from build123d import *

# Parameters (mm, degrees)
SKETCH1_W           = 101.6
SKETCH1_H           = 38.1
BOSS_EXTRUDE1_DEPTH = 38.1
BOSS_EXTRUDE2_DEPTH = 25.4
BOSS_EXTRUDE3_DEPTH = 381
SCALE1_SCALE        = 1.5


with BuildPart() as part:
    # Sketch1 → Boss-Extrude1 (new body)
    with BuildSketch(Plane(origin=(0, 0, 0), x_dir=(1, 0, 0), z_dir=(0, 1, 0))):
        with Locations((50.8, 19.05)):
            Rectangle(SKETCH1_W, SKETCH1_H)
    extrude(amount=BOSS_EXTRUDE1_DEPTH)

    # Sketch2 → Boss-Extrude2 (add)
    with BuildSketch(Plane(origin=(101.6, 0, 0), x_dir=(0, 0, -1), z_dir=(1, 0, 0))):
        with BuildLine():
            ThreePointArc((28.108587284, 28.108587284), (19.05, 31.860776993), (9.991412716, 28.108587284))
            Line((9.991412716, 28.108587284), (19.05, 19.05))
            Line((19.05, 19.05), (28.108587284, 28.108587284))
        make_face()
        with BuildLine():
            Line((19.05, 19.05), (9.991412716, 28.108587284))
            ThreePointArc((9.991412716, 28.108587284), (6.239223007, 19.05), (9.991412716, 9.991412716))
            Line((9.991412716, 9.991412716), (19.05, 19.05))
        make_face()
        with BuildLine():
            Line((28.108587284, 28.108587284), (19.05, 19.05))
            Line((19.05, 19.05), (28.108587284, 9.991412716))
            ThreePointArc((28.108587284, 9.991412716), (30.885614659, 14.147527889), (31.860776993, 19.05))
            ThreePointArc((31.860776993, 19.05), (30.885614659, 23.952472111), (28.108587284, 28.108587284))
        make_face()
        with BuildLine():
            Line((28.108587284, 9.991412716), (19.05, 19.05))
            Line((19.05, 19.05), (9.991412716, 9.991412716))
            ThreePointArc((9.991412716, 9.991412716), (19.05, 6.239223007), (28.108587284, 9.991412716))
        make_face()
    extrude(amount=BOSS_EXTRUDE2_DEPTH)

    # Sketch3 → Boss-Extrude3 (add)
    with BuildSketch(Plane(origin=(0, 38.1, 0), x_dir=(1, 0, 0), z_dir=(0, 1, 0))):
        with BuildLine():
            Line((33.415123016, 4.684876984), (19.05, 19.05))
            Line((19.05, 19.05), (4.684876984, 4.684876984))
            ThreePointArc((4.684876984, 4.684876984), (8.08545393, 1.947595257), (11.992307848, 0))
            Line((11.992307848, 0), (26.107692152, 0))
            ThreePointArc((26.107692152, 0), (30.01454607, 1.947595257), (33.415123016, 4.684876984))
        make_face()
        with BuildLine():
            Line((33.415123016, 33.415123016), (19.05, 19.05))
            Line((19.05, 19.05), (33.415123016, 4.684876984))
            ThreePointArc((33.415123016, 4.684876984), (37.818937718, 11.275651446), (39.365351794, 19.05))
            ThreePointArc((39.365351794, 19.05), (37.818937718, 26.824348554), (33.415123016, 33.415123016))
        make_face()
        with BuildLine():
            ThreePointArc((11.992307848, 38.1), (8.08545393, 36.152404743), (4.684876984, 33.415123016))
            Line((4.684876984, 33.415123016), (19.05, 19.05))
            Line((19.05, 19.05), (33.415123016, 33.415123016))
            ThreePointArc((33.415123016, 33.415123016), (30.01454607, 36.152404743), (26.107692152, 38.1))
            Line((26.107692152, 38.1), (11.992307848, 38.1))
        make_face()
        with BuildLine():
            Line((19.05, 19.05), (4.684876984, 33.415123016))
            ThreePointArc((4.684876984, 33.415123016), (1.947595257, 30.01454607), (0, 26.107692152))
            Line((0, 26.107692152), (0, 11.992307848))
            ThreePointArc((0, 11.992307848), (1.947595257, 8.08545393), (4.684876984, 4.684876984))
            Line((4.684876984, 4.684876984), (19.05, 19.05))
        make_face()
        with BuildLine():
            ThreePointArc((35.21117424, 35.21117424), (33.516839784, 36.74400046), (31.677929586, 38.1))
            Line((31.677929586, 38.1), (26.107692152, 38.1))
            ThreePointArc((26.107692152, 38.1), (30.01454607, 36.152404743), (33.415123016, 33.415123016))
            Line((33.415123016, 33.415123016), (35.21117424, 35.21117424))
        make_face()
        with BuildLine():
            ThreePointArc((41.905351794, 19.05), (40.165591731, 27.796364472), (35.21117424, 35.21117424))
            Line((35.21117424, 35.21117424), (33.415123016, 33.415123016))
            ThreePointArc((33.415123016, 33.415123016), (37.818937718, 26.824348554), (39.365351794, 19.05))
            ThreePointArc((39.365351794, 19.05), (37.818937718, 11.275651446), (33.415123016, 4.684876984))
            Line((33.415123016, 4.684876984), (35.21117424, 2.88882576))
            ThreePointArc((35.21117424, 2.88882576), (40.165591731, 10.303635528), (41.905351794, 19.05))
        make_face()
        with BuildLine():
            Line((35.21117424, 2.88882576), (33.415123016, 4.684876984))
            ThreePointArc((33.415123016, 4.684876984), (30.01454607, 1.947595257), (26.107692152, 0))
            Line((26.107692152, 0), (31.677929586, 0))
            ThreePointArc((31.677929586, 0), (33.516839784, 1.35599954), (35.21117424, 2.88882576))
        make_face()
        with BuildLine():
            Line((4.684876984, 4.684876984), (2.88882576, 2.88882576))
            ThreePointArc((2.88882576, 2.88882576), (4.583160216, 1.35599954), (6.422070414, 0))
            Line((6.422070414, 0), (11.992307848, 0))
            ThreePointArc((11.992307848, 0), (8.08545393, 1.947595257), (4.684876984, 4.684876984))
        make_face()
        with BuildLine():
            Line((0, 11.992307848), (0, 6.422070414))
            ThreePointArc((0, 6.422070414), (1.35599954, 4.583160216), (2.88882576, 2.88882576))
            Line((2.88882576, 2.88882576), (4.684876984, 4.684876984))
            ThreePointArc((4.684876984, 4.684876984), (1.947595257, 8.08545393), (0, 11.992307848))
        make_face()
        with BuildLine():
            ThreePointArc((6.422070414, 38.1), (4.583160216, 36.74400046), (2.88882576, 35.21117424))
            Line((2.88882576, 35.21117424), (4.684876984, 33.415123016))
            ThreePointArc((4.684876984, 33.415123016), (8.08545393, 36.152404743), (11.992307848, 38.1))
            Line((11.992307848, 38.1), (6.422070414, 38.1))
        make_face()
        with BuildLine():
            Line((4.684876984, 33.415123016), (2.88882576, 35.21117424))
            ThreePointArc((2.88882576, 35.21117424), (1.35599954, 33.516839784), (0, 31.677929586))
            Line((0, 31.677929586), (0, 26.107692152))
            ThreePointArc((0, 26.107692152), (1.947595257, 30.01454607), (4.684876984, 33.415123016))
        make_face()
    extrude(amount=BOSS_EXTRUDE3_DEPTH)


with BuildPart() as part_1:
    # Scale1: scaled about (28.106189099, 181.291595576, -19.05)
    add(part.part.scale(SCALE1_SCALE).moved(Location((-14.05309455, -90.645797788, 9.525))))


solid = part_1.part
Work out the finished part from the listing and answer in its coordinate system (mm). A direction names the side the tool comes from. Round coordinates to 2 decimals unless told otherwise and drop trailing zeros. Write each loop counter-clockwise with the first axis right and the second up, starting at its lowest first coordinate (ties: lowest second). Pieces come first, ordered by that corner, then holes. Notation, with made-up numbers: M 89,21.5 L 131,21.5 A24 cw 131,46.5 Z; hole C -27.75,-19.5 d8. An arc over 180 degrees is marked long. Use a Markdown table: item, result.
1) The part is cut by section D-D on x = 66. Give the vertices of the cut face in (y, z) (3 decimals), plus the area to 3 significant figures.
Taken from the geometry:
| item | result |
|---|---|
| outline | M -90.646,-47.625 L -33.496,-47.625 L -33.496,9.525 L -90.646,9.525 Z |
| area | 3,270 mm2 |
2) Flat-ended cylindrical pins translate along their axes: pin 1 (1.5 mm diameter, centred on x = 46.5, y = 277.5, fed in from -Z); pin 2 (2 mm diameter, centred on x = 36.5, y = 321, fed in from -Z); pin 3 (4 mm diameter, centred on y = -22.5, z = -33, fed in from +X). Find the tip coordinate at first contact, or state that the pin passes through.
Taken from the geometry:
| item | result |
|---|---|
| pin 1 | stops at z = -33.2 |
| pin 2 | stops at z = -46.17 |
| pin 3 | stops at x = 46.65 |
3) The part is cut by section A-A on y = 222.5. Give the vertices of the cut face in (x, z) (3 decimals), plus the area to 3 significant figures.
Taken from the geometry:
| item | result |
|---|---|
| outline | M -14.053,-37.992 A34.283 ccw -4.42,-47.625 L 33.464,-47.625 A34.283 ccw 33.464,9.525 L -4.42,9.525 A34.283 ccw -14.053,-0.108 Z |
| area | 3,250 mm2 |
4) The part is cut by section C-C on z = -25. Give the vertices of the cut face in (x, y), plus the area to 3 significant figures.
Taken from the geometry:
| item | result |
|---|---|
| outline | M -14.05,-90.65 L 138.35,-90.65 L 138.35,-80.34 L 176.45,-80.34 L 176.45,-43.8 L 138.35,-43.8 L 138.35,-33.5 L 48.28,-33.5 L 48.28,538 L -14.05,538 Z |
| area | 45,700 mm2 |
5) Consider line 1 (Y direction, x = 84, z = -13.5); line 2 (X direction, y = 409, z = -4.5); line 3 (X direction, y = 265, z = -9). Determine where each line is inside the solid, lowest interval first. Write a range as [from, to].
Taken from the geometry:
| item | result |
|---|---|
| line 1 | y = [-90.65, -33.5] |
| line 2 | x = [-14.05, 45.56] |
| line 3 | x = [-14.05, 47.3] |
6) The part is cut by section B-B on x = 156. Give the vertices of the cut face in (y, z), plus the area to 3 significant figures.
Taken from the geometry:
| item | result |
|---|---|
| outline | C -62.07,-19.05 d38.43 |
| area | 1,160 mm2 |
7) Which of the six approach directions +Z, -Z, +X, -X, +Y, -Y give full straight-line access (tool end or side, diameter ignored) to faces 1 (the face through (138.347, -82, -19)), 2 (the face through (17, 538.004, -19))?
Taken from the geometry:
| item | result |
|---|---|
| face 1 | +X |
| face 2 | +Z, -Z, +X, -X, +Y |
